Check sheet for the modelled part. Datum: model origin and axes. Units: mm. A direction names the side the tool comes from. Give positions to 0.01 mm unless a question says otherwise; leave off trailing zeros. Write each loop counter-clockwise with the first axis right and the second up, starting at its lowest first coordinate (ties: lowest second). Pieces come first, ordered by that corner, then holes. Notation, with made-up numbers: M 83,-20 L 140,-20 A34 cw 140,17 Z; hole C 78.5,-32.75 d3. An arc over 180 degrees is marked long. Write item = value, one per line. Start each with the question number.
1) Cross-section at A-A, the plane y = 28. Record the cut outline in (x, z), plus the area to 3 significant figures.
2) Access from +Z, -Z, +X, -X, +Y, -Y to the whole of each face (thin tool, end or side, straight path). Record for faces 1 (the flat face through (-2, 40, -15)), 2 (the cylindrical face through (-50.04, 29.58, -48.95)), 3 (the flat face through (-56, 40, -3.5)), 4 (the flat face through (-35, 60, -35)).
3) Cross-section at C-C, the plane x = -13. Record the cut outline in (y, z).
4) Mould release check, pull along X, two halves, no side actions. Record for faces 5 (the flat face through (0, 16, -35)), 6 (the flat face through (-14, 40, -3.5)), 7 (the flat face through (-27, 0, -27)): released by +X, released by -X, zero draft, split by the parting line, or undercut.
5) Cross-section at D-D, the plane z = -36.5. Record the cut outline in (x, y), plus the area to 3 significant figures.
6) Go/stop test with flat-tipped pins: pin 1 (20 mm diameter, centred on x = -34.5, y = 37.5, fed in from +Z); pin 2 (4 mm diameter, centred on x = -1.5, y = 36, fed in from -Z); pin 3 (1.8 mm diameter, centred on y = 46, z = -2, fed in from -X); pin 4 (5 mm diameter, centred on y = 16.5, z = -15, fed in from -X). Record where each tip stops, or that it passes through.
7) Cross-section at B-B, the plane z = -19. Record the cut outline in (x, y).
8) Scan lines: line 1 along Z through (x, y) = (-12.5, 27.5); line 2 along Z through (x, y) = (-6.5, 50); line 3 along Y through (x, z) = (-3.5, -16.5). Record each from-to range of solid material in increasing order. Write a range as [from, to].
Autodesk Inventor part; units mm, degrees
ref_plane "YZ Plane" through (0, 0, 0) normal (1, 0, 0) x (0, 1, 0)
ref_plane "XZ Plane" through (0, 0, 0) normal (0, 1, 0) x (-1, 0, 0)
ref_plane "XY Plane" through (0, 0, 0) normal (0, 0, 1) x (1, 0, 0)
sketch "Sketch1" plane through (0, 0, 0) normal (0, 1, 0) x (-1, 0, 0)
  line L0 (0, 0) -> (70, 0)
  line L1 (0, 0) -> (0, -70)
  arc A0 (0, -70) -> (70, 0) centre (0, 0) ccw
  dimension "d0" = 70
  dimension "d1" = 70
  dimension "d3" = 70
extrude "Extrusion1" add sketch "Sketch1" along normal blind 60
sketch "Sketch2" plane through (0, 0, 0) normal (1, 0, 0) x (0, 0, -1)
  line L0 (15, 60) -> (55, 60)
  line L1 (55, 60) -> (55, 20)
  line L2 (55, 20) -> (15, 20)
  line L3 (15, 20) -> (15, 60)
  line L4 (0, 60) -> (70, 60)
  line L5 (0, 0) -> (0, 60)
  dimension "d8" = 40
  dimension "d9" = 40
  dimension "d10" = 15
extrude "Extrusion2" cut sketch "Sketch2" against normal blind 7
sketch "Sketch3" plane through (-70, 0, 0) normal (0, 0, 1) x (1, 0, 0)
  line L0 (15, 60) -> (55, 60)
  line L1 (55, 60) -> (55, 20)
  line L2 (55, 20) -> (15, 20)
  line L3 (15, 20) -> (15, 60)
  line L4 (0, 60) -> (70, 60)
  line L5 (0, 0) -> (0, 60)
  point P0 (70, 0)
  point P1 (35, 20)
  point P2 (35, 60)
  dimension "d11" = 40
  dimension "d13" = 40
  dimension "d31" = 15
extrude "Extrusion3" cut sketch "Sketch3" against normal blind 7
sketch "Sketch4" plane through (0, 20, -55) normal (0, 0, 1) x (1, 0, 0)
  line L0 (-3.5, 40) -> (-7, 40)
  line L1 (-7, 40) -> (-7, 0)
  line L2 (-7, 0) -> (-3.5, 0)
  line L3 (-3.5, 0) -> (-3.5, 40)
  line L4 (0, 40) -> (0, 0)
  line L5 (-7, 40) -> (0, 40)
  line L6 (0, 0) -> (-7, 0)
  line L7 (-7, 40) -> (-7, 0)
  point P0 (0, -20)
  dimension "d16" = 3.5
extrude "Extrusion4" cut sketch "Sketch4" against normal blind 3 contours L3 L2 L1 L0
sketch "Sketch5" plane through (0, 20, -15) normal (0, 0, -1) x (-1, 0, 0)
  line L0 (3.5, 40) -> (7, 40)
  line L1 (7, 0) -> (3.5, 0)
  line L2 (3.5, 0) -> (3.5, 40)
  line L3 (3.5, 40) -> (7, 40)
  line L4 (7, 40) -> (7, 0)
  line L5 (0, 0) -> (7, 0)
  line L6 (7, 0) -> (7, 40)
  point P0 (0, -20)
  dimension "d4" = 60
  dimension "d19" = 3.5
extrude "Extrusion5" cut sketch "Sketch5" against normal blind 3
sketch "Sketch8" plane through (-15, 20, 0) normal (-1, 0, 0) x (0, 0, 1)
  line L0 (-7, 40) -> (-3.5, 40)
  line L1 (-3.5, 40) -> (-3.5, 0)
  line L2 (-3.5, 0) -> (-7, 0)
  line L3 (-7, 0) -> (-7, 40)
  line L4 (-7, 40) -> (0, 40)
  line L5 (-7, 40) -> (-7, 0)
  line L6 (0, 0) -> (-7, 0)
  point P0 (0, -20)
  dimension "d28" = 3.5
extrude "Extrusion8" cut sketch "Sketch8" against normal blind 3
sketch "Sketch9" plane through (-55, 20, 0) normal (1, 0, 0) x (0, 0, -1)
  line L0 (3.5, 40) -> (7, 40)
  line L1 (7, 40) -> (7, 0)
  line L2 (7, 0) -> (3.5, 0)
  line L3 (3.5, 0) -> (3.5, 40)
  line L4 (0, 40) -> (7, 40)
  line L5 (7, 0) -> (7, 40)
  line L6 (0, 0) -> (7, 0)
  point P0 (0, -20)
  dimension "d32" = 3.5
extrude "Extrusion9" cut sketch "Sketch9" against normal blind 3
sketch "Sketch10" plane through (0, 0, 0) normal (1, 0, 0) x (0, 0, -1)
  line L0 (0, 0) -> (0, 60)
  arc A0 (0, 2.5) -> (0, 7.5) centre (0, 5) ccw
  line L1 (70, 0) -> (0, 0)
  line L2 (0, 7.5) -> (0, 2.5)
  dimension "d35" = 5
  dimension "d36" = 5
revolve "Revolution1" cut sketch "Sketch10" angle 360 about axis through (0, 0, 0) along (0, 1, 0)
ref_plane "Work Plane1" through (0, 60, 0) normal (0.7071, 0, -0.7071) x (0, -1, 0)
sketch "Sketch11" plane through (0, 60, 0) normal (0.7071, 0, -0.7071) x (0, -1, 0)
  circle A0 centre (40, 3.5) radius 1.5
  line L0 (52.5, 0) -> (0, 0)
  line L1 (60, 49.4975) -> (60, 0)
  dimension "d38" = 3
  dimension "d41" = 3.5
  dimension "d42" = 20
extrude "Extrusion10" cut sketch "Sketch11" along normal mid plane 10
properties part number "Ecke"
Reply:
q1.outline = M -70,0 A70 ccw 0,-70 L 0,-55 L -3.5,-55 L -3.5,-58 L -7,-58 L -7,-12 L -3.5,-12 L -3.5,-15 L 0,-15 L 0,0 L -15,0 L -15,-3.5 L -12,-3.5 L -12,-7 L -58,-7 L -58,-3.5 L -55,-3.5 L -55,0 Z
q1.area = 3,250 mm2
q2.face_1 = +X, +Y
q2.face_2 = -Z, -X, +Y, -Y
q2.face_3 = +Y
q2.face_4 = +Z, -Z, +X, -X, +Y
q3.outline = M 0,-68.78 L 60,-68.78 L 60,-7 L 20,-7 L 20,-3.5 L 60,-3.5 L 60,0 L 0,0 Z
q4.face_5 = released by +X
q4.face_6 = undercut
q4.face_7 = zero draft
q5.outline = M -59.73,0 L 0,0 L 0,20 L -7,20 L -7,60 L -59.73,60 Z
q5.area = 3,300 mm2
q6.pin_1 = -7
q6.pin_2 = -70
q6.pin_3 = -69.99
q6.pin_4 = -68.87
q7.outline = M -67.37,0 L 0,0 L 0,20 L -7,20 L -7,60 L -67.37,60 Z
q8.line_1 = [-68.87, -7], [-3.5, 0]
q8.line_2 = [-69.7, -58], [-12, 0]
q8.line_3 = [0, 20]
